Autodesk Inventor part; units mm, degrees
ref_plane "YZ Plane" through (0, 0, 0) normal (1, 0, 0) x (0, 1, 0)
ref_plane "XZ Plane" through (0, 0, 0) normal (0, 1, 0) x (-1, 0, 0)
ref_plane "XY Plane" through (0, 0, 0) normal (0, 0, 1) x (1, 0, 0)
sketch "Sketch1" plane through (0, 0, 0) normal (0, 1, 0) x (-1, 0, 0)
  arc A0 (0, -7) -> (0, 7) centre (0, 0) ccw
  line L0 (0, 7) -> (0, -7)
  dimension "d0" = 14
extrude "Extrusion1" add sketch "Sketch1" along normal blind 12
ref_plane "Work Plane1" through (-10, 0, 7) normal (1, 0, 0) x (0, 0, -1)
sketch "Sketch2" plane through (-10, 0, 7) normal (1, 0, 0) x (0, 0, -1)
  line L0 (2, 8) -> (2, 1.5)
  line L1 (2, 1.5) -> (12, 1.5)
  line L2 (12, 1.5) -> (12, 7.9943)
  line L3 (9, 10.4943) -> (5, 10.4943)
  line L4 (9, 10.4943) -> (12, 7.9943)
  line L5 (5, 10.4943) -> (2, 8)
  line L6 (14, 0) -> (14, 12)
  point P0 (7, 0)
  dimension "d9" = 10
  dimension "d10" = 6.5
  dimension "d12" = 4
  dimension "d14" = 3
  dimension "d15" = 3
  dimension "d24" = 2
extrude "Extrusion2" add sketch "Sketch2" along normal blind 10
sketch "Sketch7" plane through (0, 0, 0) normal (0, 1, 0) x (-1, 0, 0)
  arc A0 (0, -7) -> (0, 7) centre (0, 0) ccw
  line L0 (0, 7) -> (0, -7)
  line L1 (0, -7) -> (0, 7)
  dimension "d40" = 7
extrude "Extrusion7" cut sketch "Sketch7" along normal through all
sketch "Sketch9" plane through (0, 0, 0) normal (0, 1, 0) x (-1, 0, 0)
  arc A0 (6.399, -5) -> (6.399, 5) centre (1.2353, 0) ccw
  arc A1 (6.399, -5) -> (6.399, 5) centre (10.7308, 0) ccw
  point P0 (0, 0)
extrude "Extrusion9" cut sketch "Sketch9" along normal through all both and the other way through all
properties part number "14mm_radius_mold_with_crystal_skull"
Source: CAD feature listing. Evaluate the final solid. Frame: model axes, mm. Give positions to 0.01 mm unless a question says otherwise; leave off trailing zeros. Write each loop counter-clockwise with the first axis right and the second up, starting at its lowest first coordinate (ties: lowest second). Pieces come first, ordered by that corner, then holes. Notation, with made-up numbers: M -0.75,-20.75 L 9.25,-20.75 A12 cw 9.25,-9.75 Z; hole C 85.5,2.5 d1. An arc over 180 degrees is marked long. Return JSON: item names as keys, results as strings. Group by question number.
1) Cut plane B-B, the plane x = -8. Output: boundary loops of the cut face in (y, z), plus the area to 3 significant figures.
2) Cut plane A-A, the plane x = -5.3. Output: boundary loops of the cut face in (y, z), plus the area to 3 significant figures.
3) Cut plane C-C, the plane z = -4. Output: boundary loops of the cut face in (x, y).
4) Material intervals for line 1 along X through (y, z) = (4.75, 2); line 2 along Z through (x, y) = (-5.25, 4); line 3 along Z through (x, y) = (-6.45, 2.5), sorted ascending. Write a range as [from, to].
5) Cut plane D-D, the plane y = 4.25. Output: boundary loops of the cut face in (x, z).
6) Pin query (flat end, axial travel): P1, Ø4, axis at y = 5.5, z = 1.5, coming from the -X side; P2, Ø2, axis at x = -7.5, y = 4.5, coming from the +Z side. Return the tip coordinate at first contact, or that it passes through.
Recorded:
{
 "1": {"outline": "M 1.5,-2.43 L 10.14,-2.43 L 10.49,-2 L 10.49,2 L 10.14,2.43 L 1.5,2.43 Z", "area": "43.6 mm²"},
 "2": {"outline": "M 1.5,-5 L 7.99,-5 L 8.35,-4.57 L 1.5,-4.57 Z; M 1.5,4.57 L 8.36,4.57 L 8,5 L 1.5,5 Z", "area": "5.70 mm²"},
 "3": {"outline": "M -7.21,1.5 L -5.74,1.5 L -5.74,8.83 L -7.21,8.83 Z"},
 "4": {"line 1": "x = [-8.14, -6.71]", "line 2": "z = [-5, -4.63], [4.63, 5]", "line 3": "z = [-4.95, -2.72], [2.72, 4.95]"},
 "5": {"outline": "M -6.4,-5 L -4.9,-5 A7 cw -4.9,5 L -6.4,5 A7.19 ccw Z"},
 "6": {"P1": "stops at x = -8.42", "P2": "stops at z = 4.89"}
}
